Can you work these out from the model? Positions are in its coordinate system, mm. Coordinates: 2 decimals unless noted, no trailing zeros. Write each loop counter-clockwise with the first axis right and the second up, starting at its lowest first coordinate (ties: lowest second). Pieces come first, ordered by that corner, then holes. Notation, with made-up numbers: (3.5, 69.25) - (34.5, 69.25) arc R20 ccw to (34.5, 78.25) - close; hole circle Ø5 at (-36.5, 49.25). An arc over 180 degrees is marked (long way). Use one line per item in the form item = value. Start each with the question number.
(1) For pin 1 Ø17.5 at (x, y) = (0, -350) entering from -Z; pin 2 Ø4 at (y, z) = (-55, 7.5) entering from +X; pin 3 Ø1.5 at (x, z) = (-201, 6) entering from +Y; pin 4 Ø4 at (y, z) = (-173, 5) entering from +X, each with a flat end and sliding along its axis, tell me the tip position at first contact or that it passes through.
(2) If I drill on probe 1 along Y at (x, z) = (0, 2); probe 2 along Y at (x, z) = (-8, -6); probe 3 along Y at (x, z) = (-235, -3.25), over which ranges is the centre line in solid material (lowest first)? Write a range as from..to.
(3) If we section it at A-A on z = 3.5: Please give me the cut outline in (x, y), then the cut area to 3 significant figures.
(4) If we section it at D-D on x = -54: Please give me the cut outline in (y, z).
(5) If we section it at C-C on y = -70: Please give me the cut outline in (x, z).
(6) If we section it at B-B on x = 0: Please give me the cut outline in (y, z).
Autodesk Inventor part; units mm, degrees
ref_plane "YZ Plane" through (0, 0, 0) normal (1, 0, 0) x (0, 1, 0)
ref_plane "XZ Plane" through (0, 0, 0) normal (0, 1, 0) x (-1, 0, 0)
ref_plane "XY Plane" through (0, 0, 0) normal (0, 0, 1) x (1, 0, 0)
sketch "Sketch1" plane through (0, 0, 0) normal (0, 0, 1) x (1, 0, 0)
  circle A0 centre (0, 0) radius 20
  circle A1 centre (0, -350) radius 11
  circle A2 centre (-235, -350) radius 11
  circle A3 centre (235, -350) radius 11
  line L0 (-233.6625, -380) -> (233.6625, -380)
  arc A4 (233.6625, -380) -> (260.9808, -323.1206) centre (233.6625, -345) ccw
  circle A5 centre (0.0008, -70) radius 11
  line L1 (70, -100) -> (-70, -100)
  line L2 (-80, -110) -> (-80, -290)
  line L3 (-70, -300) -> (70, -300)
  line L4 (80, -290) -> (80, -110)
  line L5 (80, -100) -> (-80, -300) construction
  line L6 (-80, -100) -> (80, -300) construction
  line L7 (0, 64.9697) -> (0, -492.5476)
  arc A6 (-260.9808, -323.1206) -> (-233.6625, -380) centre (-233.6625, -345) ccw
  line L8 (-80, -110) -> (-70, -100)
  line L9 (80, -110) -> (70, -100)
  line L10 (70, -300) -> (80, -290)
  line L11 (-70, -300) -> (-80, -290)
  line L12 (-260.9808, -323.1206) -> (-36.0446, 26.9405)
  arc A7 (36.0446, 26.9405) -> (-36.0446, 26.9405) centre (0, 0) ccw
  line L13 (260.9808, -323.1206) -> (36.0446, 26.9405)
  point P0 (0, -200)
  point P1 (0, -200)
  dimension "d0" = 40
  dimension "d2" = 22
  dimension "d3" = 22
  dimension "d4" = 22
  dimension "d7" = 235
  dimension "d8" = 235
  dimension "d9" = 35
  dimension "d11" = 30
  dimension "d33" = 22
  dimension "d34" = 350
  dimension "d35" = 160
  dimension "d36" = 200
  dimension "d37" = 70
  dimension "d38" = 30
  dimension "d39" = 10
  dimension "d40" = 10
  dimension "d41" = 10
  dimension "d42" = 10
  dimension "d43" = 10
  dimension "d44" = 10
  dimension "d45" = 10
  dimension "d46" = 10
  dimension "d47" = 45
extrude "Extrusion2" add sketch "Sketch1" along normal mid plane 22.22 contours A0 L7 A7 L13 A4 L0 A1 L3 L10 L4 L9 L1 A5 | A0 L7 A5 L1 L8 L2 L11 L3 A1 L0 A6 L12 A7
equation "\"d8\" = d7"
equation "\"d40\" = d39"
equation "\"d42\" = d41"
equation "\"d43\" = d41"
equation "\"d44\" = d43"
equation "\"d45\" = d41"
equation "\"d46\" = d45"
properties part number "Corpo_Suporte_4_Cabos_Modelo1"
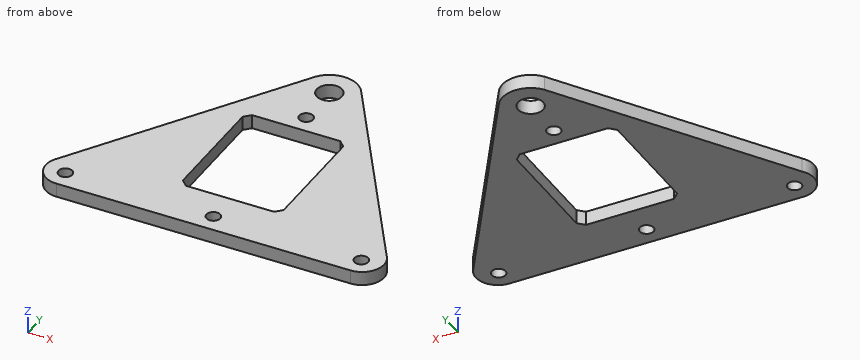
Reported:
q1.pin_1 = through
q1.pin_2 = 89.98
q1.pin_3 = -228.61
q1.pin_4 = 165.8
q2.probe_1 = -380..-361, -339..-300, -100..-81, -59..-20, 20..45
q2.probe_2 = -380..-357.55, -342.45..-300, -100..-77.55, -62.45..-18.33, 18.33..44.28
q2.probe_3 = -379.97..-361, -339..-282.69
q3.outline = (-260.98, -323.12) arc R35 ccw to (-233.66, -380) - (233.66, -380) arc R35 ccw to (260.98, -323.12) - (36.04, 26.94) arc R45 ccw to (-36.04, 26.94) - close; hole circle Ø22 at (-235, -350); hole (-80, -290) - (-70, -300) - (70, -300) - (80, -290) - (80, -110) - (70, -100) - (-70, -100) - (-80, -110) - close; hole circle Ø40 at (0, 0); hole circle Ø22 at (0, -350); hole circle Ø22 at (0, -70); hole circle Ø22 at (235, -350)
q3.area = 100,000 mm2
q4.outline = (-380, -11.11) - (-300, -11.11) - (-300, 11.11) - (-380, 11.11) - close; (-100, -11.11) - (-1, -11.11) - (-1, 11.11) - (-100, 11.11) - close
q5.outline = (-98.33, -11.11) - (-11, -11.11) - (-11, 11.11) - (-98.33, 11.11) - close; (11, -11.11) - (98.33, -11.11) - (98.33, 11.11) - (11, 11.11) - close
q6.outline = (-380, -11.11) - (-361, -11.11) - (-361, 11.11) - (-380, 11.11) - close; (-339, -11.11) - (-300, -11.11) - (-300, 11.11) - (-339, 11.11) - close; (-100, -11.11) - (-81, -11.11) - (-81, 11.11) - (-100, 11.11) - close; (-59, -11.11) - (-20, -11.11) - (-20, 11.11) - (-59, 11.11) - close; (20, -11.11) - (45, -11.11) - (45, 11.11) - (20, 11.11) - close
